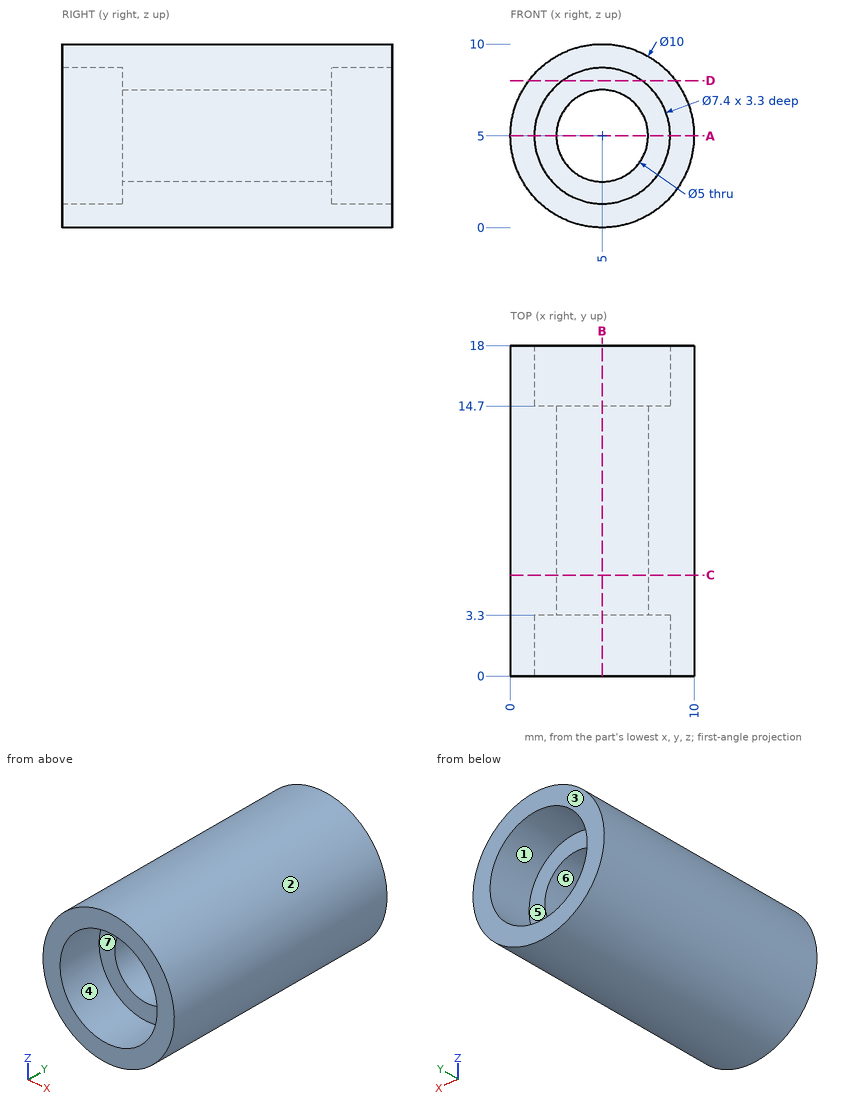
Job drawing, mm, ordinate dimensions from the low corner. One solid piece. A direction names the side the tool comes from. Round coordinates to 2 decimals unless told otherwise and drop trailing zeros. Write each loop counter-clockwise with the first axis right and the second up, starting at its lowest first coordinate (ties: lowest second). Pieces come first, ordered by that corner, then holes. Notation, with made-up numbers: (50, 81.25) -> (54, 81.25) arc R19 ccw to (54, 94.25) -> close; hole circle Ø1 at (-9, 23). An arc over 180 degrees is marked (long way). Answer as a JSON object with one key per item and string values.
(1) Two-plate mould, pull along Z, no slides. Class the marked faces 1, 2, 3 and 4: +Z half, -Z half, draft (parallel to the pull), parting line (faces both ways), or undercut.
Reported:
{"face 1": "undercut", "face 2": "parting line", "face 3": "draft", "face 4": "undercut"}
(2) Pin check, flat tips, straight feed: P1, Ø3.5, axis at x = 6, z = 5, coming from the +Y side; P2, Ø6, axis at x = 4.5, z = 8, coming from the +Y side; P3, Ø1, axis at x = 7, y = 12.5, coming from the -Z side; P4, Ø2, axis at x = 3.5, y = 3, coming from the +Z side. Stop position of each tip, or through.
Reported:
{"P1": "stops at y = 14.7", "P2": "stops at y = 18", "P3": "stops at z = 0.23", "P4": "stops at z = 9.97"}
(3) Band-saw the part on C-C, the plane y = 5.5. List the corners of the cut face in (x, z), then the cut area to 3 significant figures.
Reported:
{"outline": "circle Ø10 at (5, 5); hole circle Ø5 at (5, 5)", "area": "58.9 mm^2"}
(4) Probe probe 1 along X at (y, z) = (10, 5); probe 2 along X at (y, z) = (16.2, 5); probe 3 along Y at (x, z) = (7.25, 3.25). List the from-to ranges inside material, lowest first. Write a range as [from, to].
Reported:
{"probe 1": "x = [0, 2.5], [7.5, 10]", "probe 2": "x = [0, 1.3], [8.7, 10]", "probe 3": "y = [3.3, 14.7]"}
(5) Band-saw the part on A-A, the plane z = 5. List the corners of the cut face in (x, y).
Reported:
{"outline": "(0, 0) -> (1.3, 0) -> (1.3, 3.3) -> (2.5, 3.3) -> (2.5, 14.7) -> (1.3, 14.7) -> (1.3, 18) -> (0, 18) -> close; (7.5, 3.3) -> (8.7, 3.3) -> (8.7, 0) -> (10, 0) -> (10, 18) -> (8.7, 18) -> (8.7, 14.7) -> (7.5, 14.7) -> close"}
(6) Which spindle directions (+Z, -Z, +X, -X, +Y, -Y) get a long thin tool onto all of the face, cutting with end or side? Do the marked faces 5, 6 and 7. Say none if no direction does.
Reported:
{"face 5": "+Y", "face 6": "+Y, -Y", "face 7": "-Y"}
(7) Band-saw the part on B-B, the plane x = 5. List the corners of the cut face in (y, z).
Reported:
{"outline": "(0, 0) -> (18, 0) -> (18, 1.3) -> (14.7, 1.3) -> (14.7, 2.5) -> (3.3, 2.5) -> (3.3, 1.3) -> (0, 1.3) -> close; (0, 8.7) -> (3.3, 8.7) -> (3.3, 7.5) -> (14.7, 7.5) -> (14.7, 8.7) -> (18, 8.7) -> (18, 10) -> (0, 10) -> close"}
(8) Band-saw the part on D-D, the plane z = 8. List the corners of the cut face in (x, y).
Reported:
{"outline": "(1, 0) -> (2.83, 0) -> (2.83, 3.3) -> (7.17, 3.3) -> (7.17, 0) -> (9, 0) -> (9, 18) -> (7.17, 18) -> (7.17, 14.7) -> (2.83, 14.7) -> (2.83, 18) -> (1, 18) -> close"}
